from build123d import *

# Parameters (mm, degrees)
F0_W        = 142.3350870609
F0_H        = 111.8143312633
F1_DEPTH    = 65.532
F2_T1_DEPTH = 521.5375533391
F4_DEPTH    = 20.828
F3_W        = 65.6352208462
F3_H        = 63.7141903862
F3_W_2      = 63.7141834013
F3_H_2      = 64.0343613923
F3_W_3      = 30.4163205437
F3_H_3      = 29.4558089226
F3_W_4      = 22.0918541308
F3_H_4      = 29.1356351227
F3_W_5      = 14.0875652432
F3_W_6      = 11.8463523686
F3_W_7      = 40.6618192792
F5_DEPTH    = 72.39


# Not quite as in the source:
# - a fillet or chamfer that OpenCascade refuses, or shapes differently, is made with other operations: its cross-section is extruded or revolved along the edge and cut away or added


with BuildPart() as f1:
    # F0 (on Top) → F1 (new body)
    with BuildSketch(Plane.XY):
        with Locations((-0.4278570414, 0.1426208764)):
            Rectangle(F0_W, F0_H)
    extrude(amount=F1_DEPTH)

    # F2: fillet of radius 76.6512806053 on 1 edges, made by hand

    # F2_s2 → F2_t1 (cut)
    with BuildSketch(Plane.YZ.offset(-261.1966337109)):
        with BuildLine():
            ThreePointArc((-55.7645447552, 0), (-30.0394768726, 46.8795379871), (20.0759485004, 65.532))
            Line((20.0759485004, 65.532), (-55.7645447552, 65.532))
            Line((-55.7645447552, 65.532), (-55.7645447552, 0))
        make_face()
    extrude(amount=F2_T1_DEPTH, mode=Mode.SUBTRACT)

    # F4 (add): a face of the model
    f4_faces = [f1.faces().sort_by_distance(p)[0] for p in [
        (-0.4278570414, 0.1426208764, 0),
    ]]
    extrude(f4_faces, amount=F4_DEPTH)

    # F3 (on face) → F5 (cut)
    with BuildSketch(Plane.XY.offset(65.532)):
        with Locations((-36.3275922136, -17.8819601424)):
            Rectangle(F3_W, F3_H)
        with Locations((34.7505474929, -17.7218746394)):
            Rectangle(F3_W_2, F3_H_2)
        with Locations((18.1016160641, 38.6283630505)):
            Rectangle(F3_W_3, F3_H_3)
        with Locations((-14.555908856, 38.4682761505)):
            Rectangle(F3_W_4, F3_H_4)
        with Locations((43.5552746058, 38.4682761505)):
            Rectangle(F3_W_5, F3_H_4)
        with Locations((60.6844630092, 38.4682761505)):
            Rectangle(F3_W_6, F3_H_4)
        with Locations((-48.8142929971, 38.4682761505)):
            Rectangle(F3_W_7, F3_H_4)
    extrude(amount=-F5_DEPTH, mode=Mode.SUBTRACT)


solid = f1.part
Geometry check sheet. Reference: the model listing, model coordinates, mm. Round coordinates to 2 decimals unless told otherwise and drop trailing zeros. Loops run counter-clockwise (first coordinate to the right, second up) from the corner with the lowest first, then second, coordinate; pieces in that order, holes last.
Item 1: Mould release check, pull along Y, two halves, no side actions. Record for faces 1 (the flat face through (-37, -49.739, 7)), 2 (the flat face through (-71.595, -1, 23)): pulls with the +Y half, pulls with the -Y half, needs draft (parallel to the pull), parting line crosses it, or undercut.
Item 2: Cross-section at B-B on x = -14. Record the boundary of the cut face in (y, z), then the cut area to 3 significant figures.
Item 3: Cross-section at A-A on y = 45. Record the boundary of the cut face in (x, z).
Item 4: Gauge pin test, flat ends, axial feed: pin 1 (6.5 mm diameter, centred on x = -19.5, z = 21.5, fed in from -Y); pin 2 (4 mm diameter, centred on x = 42.5, z = 21, fed in from -Y); pin 3 (14.5 mm diameter, centred on x = 21, y = 38, fed in from +Z). Record the tip position at first contact, or that the pin passes through.
Item 5: Thickness scan on line 1 (X direction, y = 40.5, z = 37); line 2 (Y direction, x = 8, z = -4); line 3 (X direction, y = 1, z = 2). Record the ranges inside material, lowest first.
Item 6: Cross-section at C-C on z = 8.5. Count the separate pieces of the cut face and the enclosed holes in it, then the cut area to 3 significant figures.
Answer sheet:
1. face 1: undercut
1. face 2: needs draft
2. outline: (-55.76, -20.83) - (56.05, -20.83) - (56.05, 65.53) - (53.04, 65.53) - (53.04, -6.86) - (23.9, -6.86) - (23.9, 65.53) - (20.08, 65.53) arc R76.65 ccw to (13.98, 65.29) - (13.98, -6.86) - (-49.74, -6.86) - (-49.74, 20.52) arc R76.65 ccw to (-55.76, 0) - close
2. area: 2,610 mm2
3. outline: (-71.6, -20.83) - (70.74, -20.83) - (70.74, 65.53) - (66.61, 65.53) - (66.61, -6.86) - (54.76, -6.86) - (54.76, 65.53) - (50.6, 65.53) - (50.6, -6.86) - (36.51, -6.86) - (36.51, 65.53) - (33.31, 65.53) - (33.31, -6.86) - (2.89, -6.86) - (2.89, 65.53) - (-3.51, 65.53) - (-3.51, -6.86) - (-25.6, -6.86) - (-25.6, 65.53) - (-28.48, 65.53) - (-28.48, -6.86) - (-69.15, -6.86) - (-69.15, 65.53) - (-71.6, 65.53) - close
4. pin 1: stops at y = -50.73
4. pin 2: stops at y = -50.41
4. pin 3: stops at z = -6.86
5. line 1: x = -71.6 to -69.15, -28.48 to -25.6, -3.51 to 2.89, 33.31 to 36.51, 50.6 to 54.76, 66.61 to 70.74
5. line 2: y = -55.76 to -49.74, 14.3 to 23.9, 53.36 to 56.05
5. line 3: x = -71.6 to -69.15, -3.51 to 2.89, 66.61 to 70.74
6. separate pieces: 1
6. enclosed holes: 7
6. area: 3,930 mm2
